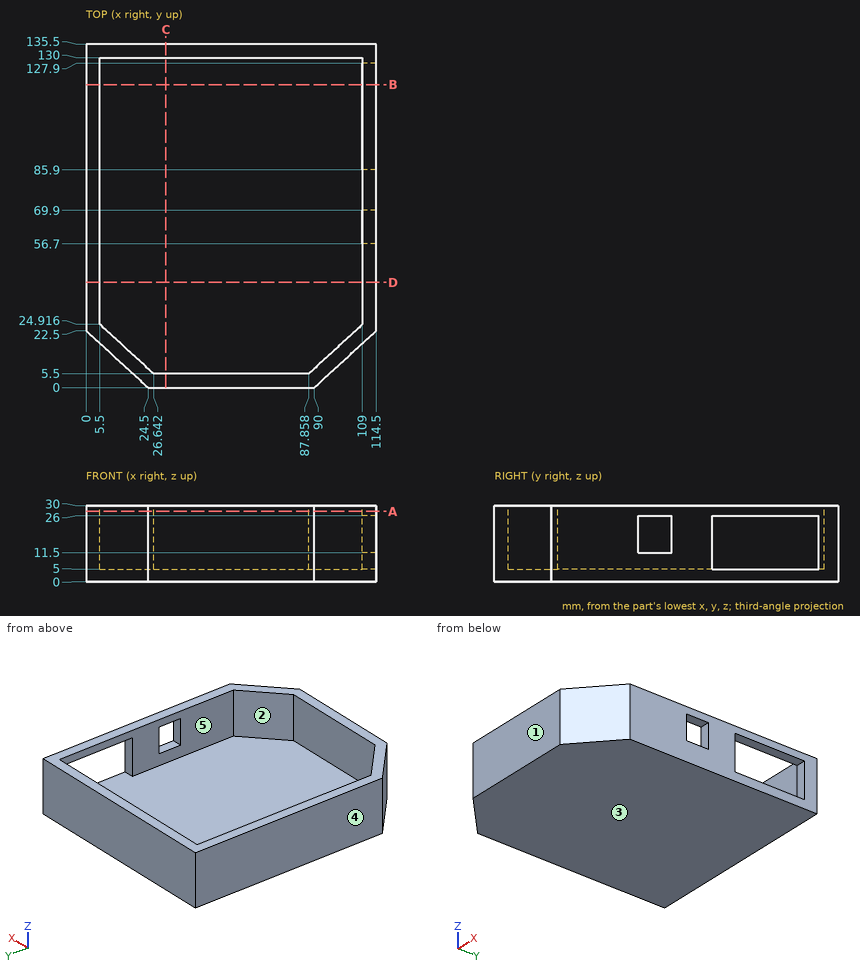
The figure shows three views and two pictorial views of one solid part (mm, origin at its lowest corner). Answer the questions. A direction names the side the tool comes from. Coordinates: 2 decimals unless noted, no trailing zeros. Loops run counter-clockwise (first coordinate to the right, second up) from the corner with the lowest first, then second, coordinate; pieces in that order, holes last. Notation, with made-up numbers: (23, -10) -> (30, -10) arc R34 ccw to (30, 27) -> close; hole circle Ø2 at (-32.75, 36.25). An arc over 180 degrees is marked (long way). Write item = value, one per line. Start each with the question number.
1) A cutting plane is placed at C-C (x = 31.5). Give the vertices of the cut face in (y, z).
2) Given pin 1 Ø12 at (x, y) = (28.5, 65) entering from +Z; pin 2 Ø3 at (x, z) = (113, 22) entering from -Y (1 decimal); pin 3 Ø3 at (x, z) = (111, 17) entering from -Y, each flat-ended and moving along its own axis, determine where each tip first touches the part or whether it passes through.
3) The mould has two halves that part along Y. Classify the marked faces 1, 2 and 3: released by +Y, released by -Y, zero draft, split by the parting line, or undercut.
4) A cutting plane is placed at D-D (y = 41.5). Give the vertices of the cut face in (x, z).
5) A tool of negligible diameter and unlimited length cuts with its end or side. For the marked faces 4 and 5, from which of +Z, -Z, +X, -X, +Y, -Y can it reach the whole face along a straight path? Write none if from no direction.
6) A cutting plane is placed at B-B (y = 119.5). Give the vertices of the cut face in (x, z).
7) Straight lines are drawn through the part: line 1 (X direction, y = 37.5, z = 24.5); line 2 (Y direction, x = 43.5, z = 27); line 3 (Z direction, x = 59.5, y = 92.5). For each, find the intervals that lie inside material, in ascending order. Write a range as from..to.
8) A cutting plane is placed at A-A (z = 27.75). Give the vertices of the cut face in (x, y), then the cut area to 3 significant figures.
Responses:
q1.outline = (0, 0) -> (135.5, 0) -> (135.5, 30) -> (130, 30) -> (130, 5) -> (5.5, 5) -> (5.5, 30) -> (0, 30) -> close
q2.pin_1 = 5
q2.pin_2 = 19.7
q2.pin_3 = 17.91
q3.face_1 = released by -Y
q3.face_2 = undercut
q3.face_3 = zero draft
q4.outline = (0, 0) -> (114.5, 0) -> (114.5, 30) -> (109, 30) -> (109, 5) -> (5.5, 5) -> (5.5, 30) -> (0, 30) -> close
q5.face_4 = +Z, -Z, -X, +Y, -Y
q5.face_5 = +Z
q6.outline = (0, 0) -> (114.5, 0) -> (114.5, 5) -> (5.5, 5) -> (5.5, 30) -> (0, 30) -> close; (109, 26) -> (114.5, 26) -> (114.5, 30) -> (109, 30) -> close
q7.line_1 = 0..5.5, 109..114.5
q7.line_2 = 0..5.5, 130..135.5
q7.line_3 = 0..5
q8.outline = (0, 22.5) -> (24.5, 0) -> (90, 0) -> (114.5, 22.5) -> (114.5, 135.5) -> (0, 135.5) -> close; hole (5.5, 24.92) -> (26.64, 5.5) -> (87.86, 5.5) -> (109, 24.92) -> (109, 130) -> (5.5, 130) -> close
q8.area = 2,490 mm²
